Could you check a few things on this model? Use its own coordinates, in mm. Face numbers are marked on the shaded views. A direction names the side the tool comes from. Give positions to 0.01 mm unless a question says otherwise; leave off trailing zeros. Order: outer loops, then holes, each group sorted by start corner. A loop starts at its lowest first (then second) coordinate and runs counter-clockwise, first axis right, second up. Notation, with made-up numbers: (55.25, -30) -> (61.25, -30) arc R22 ccw to (61.25, 8) -> close; hole circle Ø10 at (7, 23). An arc over 180 degrees is marked (long way). Use one line per item in the form item = value. Start each with the question number.
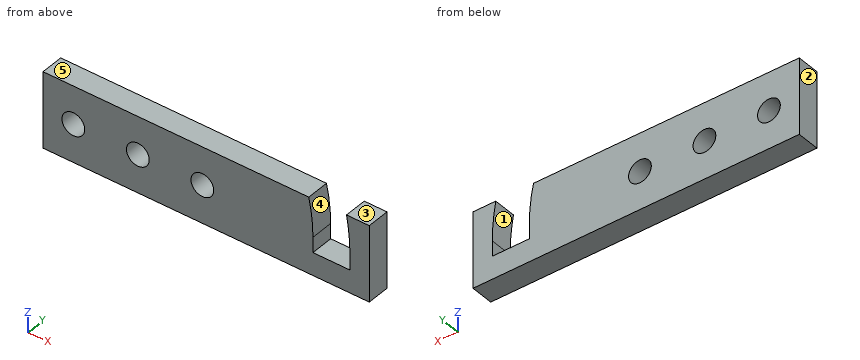
from build123d import *

# Parameters (mm, degrees)
ESQUISSE1_R             = 1.5
BOSS_EXTRU_2_DEPTH      = 3
ENL_V_MAT_EXTRU_2_DEPTH = 3
ESQUISSE3_W             = 4.875673512
ESQUISSE3_H             = 2
ENL_V_MAT_EXTRU_3_DEPTH = 3


with BuildPart() as part:
    # Esquisse1 → Boss.-Extru.2 (new body)
    with BuildSketch(Plane(origin=(0, 0, 0), x_dir=(1, 0, 0), z_dir=(0, 1, 0))):
        Polygon((0, 0), (36.5, 0), (36.5, 2.820303555), (40, 2.820303555), (40, 0), (43, 0), (43, 10), (0, 10), align=None)
        with Locations((4, 4.99734883)):
            Circle(ESQUISSE1_R, mode=Mode.SUBTRACT)
        with Locations((12.5, 4.99734883)):
            Circle(ESQUISSE1_R, mode=Mode.SUBTRACT)
        with Locations((21, 4.99734883)):
            Circle(ESQUISSE1_R, mode=Mode.SUBTRACT)
    extrude(amount=BOSS_EXTRU_2_DEPTH)

    # Esquisse2 → Enlèv. mat.-Extru.2 (cut)
    with BuildSketch(Plane(origin=(0, 3, 0), x_dir=(1, 0, 0), z_dir=(0, 1, 0))):
        with BuildLine():
            Line((35.602803426, 4.99734883), (40.450375585, 4.99734883))
            ThreePointArc((40.450375585, 4.99734883), (40.337553987, 2.488547647), (40, 0))
            Line((40, 0), (40, 2.820303555))
            Line((40, 2.820303555), (36.5, 2.820303555))
            Line((36.5, 2.820303555), (36.5, 0))
            Line((36.5, 0), (35.02705885, 0))
            ThreePointArc((35.02705885, 0), (35.437382668, 2.483715582), (35.574702073, 4.99734883))
            Line((35.574702073, 4.99734883), (35.602803426, 4.99734883))
        make_face()
    extrude(amount=-ENL_V_MAT_EXTRU_2_DEPTH, mode=Mode.SUBTRACT)

    # Esquisse3 → Enlèv. mat.-Extru.3 (cut)
    with BuildSketch(Plane(origin=(0, 3, 0), x_dir=(1, 0, 0), z_dir=(0, 1, 0))):
        with Locations((38.012538829, 5.99734883)):
            Rectangle(ESQUISSE3_W, ESQUISSE3_H)
    extrude(amount=-ENL_V_MAT_EXTRU_3_DEPTH, mode=Mode.SUBTRACT)


solid = part.part
(1) Imagine slicing it at A-A (y = 1.8). Write out the boundary of the cut face in (x, z).
(2) Imagine slicing it at B-B (x = 4). Write out the boundary of the cut face in (y, z), plus the area to 3 significant figures.
(3) Please list where these lines run through material, in increasing order: probe 1 along X at (y, z) = (0.35, -4.75); probe 2 along Z at (x, y) = (4, 1.35).
(4) Which directions (+Z, -Z, +X, -X, +Y, -Y) give clear straight access to the entire face, cutting with the end or side of a thin tool? Please do the marked faces 4 and 5.
(5) Imagine slicing it at C-C (z = -2). Write out the boundary of the cut face in (x, y), plus the area to 3 significant figures.
(6) We'd pull the mould along X, two halves only. Please class the marked faces 1, 2 and 3: pulls with the +X half, pulls with the -X half, needs draft (parallel to the pull), parting line crosses it, or undercut.
Calculated:
q1.outline = (0, -10) -> (43, -10) -> (43, 0) -> (40, 0) arc R27.95 cw to (40.45, -5) -> (40.45, -7) -> (35.57, -7) -> (35.57, -5) arc R23.07 ccw to (35.03, 0) -> (0, 0) -> close; hole circle Ø3 at (4, -5); hole circle Ø3 at (12.5, -5); hole circle Ø3 at (21, -5)
q2.outline = (0, -10) -> (3, -10) -> (3, -6.5) -> (0, -6.5) -> close; (0, -3.5) -> (3, -3.5) -> (3, 0) -> (0, 0) -> close
q2.area = 21.0 mm2
q3.probe_1 = 0 to 2.52, 5.48 to 11.02, 13.98 to 19.52, 22.48 to 35.57, 40.45 to 43
q3.probe_2 = -10 to -6.5, -3.5 to 0
q4.face_4 = +Z, +Y, -Y
q4.face_5 = +Z, +X, -X, +Y, -Y
q5.outline = (0, 0) -> (35.38, 0) -> (35.38, 3) -> (0, 3) -> close; (40.29, 0) -> (43, 0) -> (43, 3) -> (40.29, 3) -> close
q5.area = 114 mm2
q6.face_1 = undercut
q6.face_2 = pulls with the -X half
q6.face_3 = needs draft
